For this review, take the finished solid that the model builds, in its own axes (mm). Face numbers are marked on the shaded views. A direction names the side the tool comes from. Coordinates: 2 decimals unless noted, no trailing zeros. Loops run counter-clockwise (first coordinate to the right, second up) from the corner with the lowest first, then second, coordinate; pieces in that order, holes last. Notation, with made-up numbers: M 59.5,36.5 L 112.5,36.5 A18 cw 112.5,68.5 Z; hole C -27,74.5 d5. An arc over 180 degrees is marked long. Write item = value, one per line.
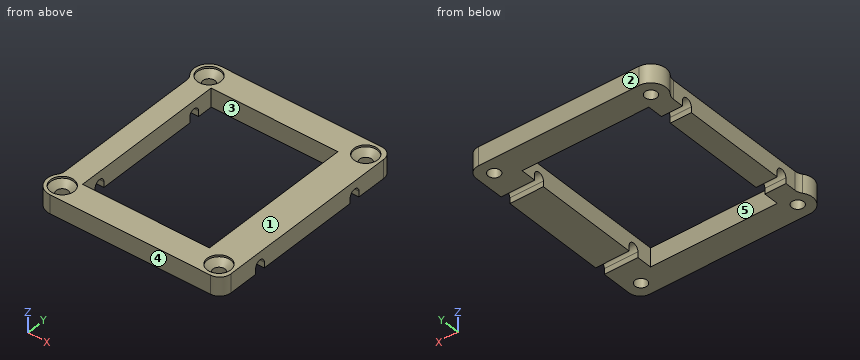
from build123d import *

# Parameters (mm, degrees)
SKETCH1_R                                    = 1.25
SKETCH1_W                                    = 36
SKETCH1_H                                    = 42.1
BOSS_EXTRUDE1_DEPTH                          = 5
SKETCH6_W                                    = 2
SKETCH6_H                                    = 42.1
BOSS_EXTRUDE4_DEPTH                          = 5
CSK_FOR_M3_COUNTERSUNK_FLAT_HEAD_SCR_2_COUNT = 2
CSK_FOR_M3_COUNTERSUNK_FLAT_HEAD_SCR_2_PITCH = 48.1
CSK_FOR_M3_COUNTERSUNK_FLAT_HEAD_SCR_3_COUNT = 2
CSK_FOR_M3_COUNTERSUNK_FLAT_HEAD_SCR_3_PITCH = 63.856166499
CSK_FOR_M3_COUNTERSUNK_FLAT_HEAD_SCR_4_COUNT = 2
CSK_FOR_M3_COUNTERSUNK_FLAT_HEAD_SCR_4_PITCH = 42
FURO_COM_FOLGA_DE_M34_D                      = 2.87
FILETE1_R                                    = 3
ESBO_O3_W                                    = 1.5
ESBO_O3_H                                    = 2.87
CORTE_EXTRUS_O1_DEPTH                        = 63
CORTE_EXTRUS_O1_DEPTH_BACK                   = 10


with BuildPart() as part:
    # Sketch1 → Boss-Extrude1 (new body)
    with BuildSketch(Plane.XY):
        with BuildLine():
            Line((20.053938932, -66.638943184), (63.053938932, -66.638943184))
            ThreePointArc((63.053938932, -66.638943184), (65.175259276, -67.517622841), (66.053938932, -69.638943184))
            Line((66.053938932, -69.638943184), (66.053938932, -119.738943184))
            ThreePointArc((66.053938932, -119.738943184), (65.175259276, -121.860263528), (63.053938932, -122.738943184))
            Line((63.053938932, -122.738943184), (20.053938932, -122.738943184))
            ThreePointArc((20.053938932, -122.738943184), (16.310928808, -120.149572552), (17.413938931, -115.73388079))
            Line((17.413938931, -115.73388079), (17.413938931, -73.644005579))
            ThreePointArc((17.413938931, -73.644005579), (16.310928808, -69.228313817), (20.053938932, -66.638943184))
        make_face()
        with Locations((20.053938932, -70.638943184)):
            Circle(SKETCH1_R, mode=Mode.SUBTRACT)
        with Locations((20.053938932, -118.738943184)):
            Circle(SKETCH1_R, mode=Mode.SUBTRACT)
        with Locations((62.053938932, -70.638943184)):
            Circle(SKETCH1_R, mode=Mode.SUBTRACT)
        with Locations((62.053938932, -118.738943184)):
            Circle(SKETCH1_R, mode=Mode.SUBTRACT)
        with Locations((41.053938932, -94.688943184)):
            Rectangle(SKETCH1_W, SKETCH1_H, mode=Mode.SUBTRACT)
    extrude(amount=BOSS_EXTRUDE1_DEPTH)

    # Sketch6 → Boss-Extrude4 (add)
    with BuildSketch(Plane.XY.offset(5)):
        with Locations((58.053938932, -94.688943184)):
            Rectangle(SKETCH6_W, SKETCH6_H)
    extrude(amount=-BOSS_EXTRUDE4_DEPTH)

    # Sketch2 → CSK for M3 Countersunk Flat Head Screw1 (revolve, cut)
    with BuildSketch(Plane(origin=(20.053938932, -118.738943184, 5), x_dir=(0, -1, 0), z_dir=(1, 0, 0))):
        Polygon((0, 0), (0, 5), (1.6, 5), (1.6, 2.05), (3.15, 0.5), (3.15, 0), align=None)
    csk_for_m3_countersunk_flat_head_screw1 = revolve(axis=Axis((20.053938932, -118.738943184, 11.35), (0, 0, -1)), mode=Mode.SUBTRACT)

    # CSK for M3 Countersunk Flat Head Scr 2: CSK for M3 Countersunk Flat Head Screw1 ×2
    with Locations(*[(0, i * CSK_FOR_M3_COUNTERSUNK_FLAT_HEAD_SCR_2_PITCH, 0) for i in range(1, CSK_FOR_M3_COUNTERSUNK_FLAT_HEAD_SCR_2_COUNT)]):
        add(csk_for_m3_countersunk_flat_head_screw1, mode=Mode.SUBTRACT)

    # CSK for M3 Countersunk Flat Head Scr 3: CSK for M3 Countersunk Flat Head Screw1 ×2
    with Locations(*[Vector(0.657728177, 0.753255365, 0) * (i * CSK_FOR_M3_COUNTERSUNK_FLAT_HEAD_SCR_3_PITCH) for i in range(1, CSK_FOR_M3_COUNTERSUNK_FLAT_HEAD_SCR_3_COUNT)]):
        add(csk_for_m3_countersunk_flat_head_screw1, mode=Mode.SUBTRACT)

    # CSK for M3 Countersunk Flat Head Scr 4: CSK for M3 Countersunk Flat Head Screw1 ×2
    with Locations(*[(i * CSK_FOR_M3_COUNTERSUNK_FLAT_HEAD_SCR_4_PITCH, 0, 0) for i in range(1, CSK_FOR_M3_COUNTERSUNK_FLAT_HEAD_SCR_4_COUNT)]):
        add(csk_for_m3_countersunk_flat_head_screw1, mode=Mode.SUBTRACT)

    # Furo com folga de M34 (through all)
    with Locations(Plane(origin=(66.053938932, 0, 0), x_dir=(0, 0, -1), z_dir=(1, 0, 0))):
        with Locations((-1.5, -79.188943184), (-1.5, -110.188943184)):
            Hole(FURO_COM_FOLGA_DE_M34_D / 2)

    # Filete1
    filete1_edges = [part.edges().sort_by_distance(p)[0] for p in [
        (17.413938931, -115.73388079, 2.5),
        (17.413938931, -73.644005579, 2.5),
    ]]
    fillet(filete1_edges, radius=FILETE1_R)

    # Esboço3 → Corte-extrusão1 (cut, two sides)
    with BuildSketch(Plane.ZY.offset(-57.053938932)) as corte_extrus_o1_sk:
        with Locations((0.75, -79.188943184)):
            Rectangle(ESBO_O3_W, ESBO_O3_H)
        with Locations((0.75, -110.188943184)):
            Rectangle(ESBO_O3_W, ESBO_O3_H)
    extrude(amount=CORTE_EXTRUS_O1_DEPTH, mode=Mode.SUBTRACT)
    extrude(corte_extrus_o1_sk.sketch, amount=-CORTE_EXTRUS_O1_DEPTH_BACK, mode=Mode.SUBTRACT)


solid = part.part
Q1. Machinability: for the marked faces 4 and 5, which of the approach directions +Z, -Z, +X, -X, +Y, -Y give a long, thin tool a straight path to every point of the face, cutting with its end or side? Answer none if there is none.
Solved:
face_4 = +Z, -Z, +X, -X, -Y
face_5 = +Z, -Z
Q2. For pin 1 Ø3 at (y, z) = (-98, 3) entering from -X; pin 2 Ø1.5 at (x, y) = (58, -77.5) entering from -Z; pin 3 Ø1 at (x, y) = (57.5, -78.5) entering from -Z, all flat-tipped, find the tip position at first contact; note any pin that passes through.
Solved:
pin_1 = 17.41
pin_2 = 0
pin_3 = 2.3
Q3. Add section B-B (y = -87). Write out the cut boundary in (x, z).
Solved:
outline = M 17.41,0 L 23.05,0 L 23.05,5 L 17.41,5 Z; M 57.05,0 L 66.05,0 L 66.05,5 L 57.05,5 Z
Q4. Add section A-A (x = 55). Write out the cut boundary in (y, z).
Solved:
outline = M -122.74,0 L -115.74,0 L -115.74,5 L -122.74,5 Z; M -73.64,0 L -66.64,0 L -66.64,5 L -73.64,5 Z
Q5. Draft analysis for pull direction Y (two halves, no side actions). For the marked faces 1, 2 and 3, state which applies: +Y half, -Y half, draft (parallel to the pull), parting line (faces both ways), or undercut.
Solved:
face_1 = draft
face_2 = +Y half
face_3 = undercut
Q6. Add section C-C (z = 3.7). Write out the cut boundary in (x, y), and give its area (3 significant figures).
Solved:
outline = M 16.83,-116.37 A4 ccw 20.05,-122.74 L 63.05,-122.74 A3 ccw 66.05,-119.74 L 66.05,-69.64 A3 ccw 63.05,-66.64 L 20.05,-66.64 A4 ccw 16.83,-73.01 A3 cw 17.41,-74.79 L 17.41,-114.59 A3 cw Z; hole C 20.05,-118.74 d4.7; hole C 20.05,-70.64 d4.7; hole M 23.05,-115.74 L 57.05,-115.74 L 57.05,-73.64 L 23.05,-73.64 Z; hole C 62.05,-118.74 d4.7; hole C 62.05,-70.64 d4.7
area = 1,230 mm²
Q7. Add section D-D (y = -118). State how many separate pieces and enclosed holes the cut face has, and give its area (3 significant figures).
Solved:
separate_pieces = 3
enclosed_holes = 0
area = 213 mm²
Q8. For line 1 along X through (y, z) = (-82, 2.95); line 2 along Y through (x, z) = (47.5, 4.25); line 3 along Y through (x, z) = (60.5, 3.6), list the stretches that pass through material, from the lowest coordinate up.
Solved:
line_1 = 17.41 to 23.05, 57.05 to 66.05
line_2 = -122.74 to -115.74, -73.64 to -66.64
line_3 = -122.74 to -120.37, -117.11 to -72.27, -69.01 to -66.64
